Could you check a few things on this model? Use its own coordinates, in mm. Coordinates: 2 decimals unless noted, no trailing zeros. Loops run counter-clockwise (first coordinate to the right, second up) from the corner with the lowest first, then second, coordinate; pieces in that order, holes last. Notation, with made-up numbers: (-25.5, 85) -> (-14.5, 85) arc R6 ccw to (-14.5, 89) -> close; hole circle Ø8 at (-15.75, 24). An arc over 180 degrees is marked (long way). One line per question, with ' | ' between items.
from build123d import *

# Parameters (mm, degrees)
SKETCH1_W               = 48.3
SKETCH1_H               = 44
SKETCH1_R               = 1.6
SKETCH1_R_2             = 2.5527
BOSS_EXTRUDE1_DEPTH     = 6.35
F_1_4_20_TAPPED_HOLE1_D = 5.1054


with BuildPart() as part:
    # Sketch1 → Boss-Extrude1 (new body)
    with BuildSketch(Plane.XY):
        with Locations((24.15, -22)):
            Rectangle(SKETCH1_W, SKETCH1_H)
        with Locations((7.5, -37)):
            Circle(SKETCH1_R, mode=Mode.SUBTRACT)
        with Locations((22.5, -9.3)):
            Circle(SKETCH1_R_2, mode=Mode.SUBTRACT)
        with Locations((35.2, -22)):
            Circle(SKETCH1_R_2, mode=Mode.SUBTRACT)
        with Locations((9.8, -22)):
            Circle(SKETCH1_R_2, mode=Mode.SUBTRACT)
        with Locations((22.5, -34.7)):
            Circle(SKETCH1_R_2, mode=Mode.SUBTRACT)
        with Locations((37.5, -37)):
            Circle(SKETCH1_R, mode=Mode.SUBTRACT)
        with Locations((37.5, -7)):
            Circle(SKETCH1_R, mode=Mode.SUBTRACT)
        with Locations((7.5, -7)):
            Circle(SKETCH1_R, mode=Mode.SUBTRACT)
    extrude(amount=BOSS_EXTRUDE1_DEPTH)

    # 1/4-20 Tapped Hole1 (through all)
    with Locations(Plane(origin=(22.5, -9.3, 6.35), x_dir=(1, 0, 0), z_dir=(0, 0, 1))):
        with Locations((0, 0), (12.7, -12.7), (-12.7, -12.7), (0, -25.4)):
            Hole(F_1_4_20_TAPPED_HOLE1_D / 2)


solid = part.part
1) We'd pull the mould along Z, two halves only. Please class faces 1 (the face through (24, -22, 6.35)), 2 (the face through (24, -22, 0)), 3 (the face through (37.15, -8.56, 3.13)): pulls with the +Z half, pulls with the -Z half, needs draft (parallel to the pull), parting line crosses it, or undercut.
Data:
face 1: pulls with the +Z half | face 2: pulls with the -Z half | face 3: needs draft
2) If we section it at A-A on x = 22.5: Please give me the cut outline in (y, z), and give its area (3 significant figures).
Data:
outline: (-44, 0) -> (-37.25, 0) -> (-37.25, 6.35) -> (-44, 6.35) -> close; (-32.15, 0) -> (-11.85, 0) -> (-11.85, 6.35) -> (-32.15, 6.35) -> close; (-6.75, 0) -> (0, 0) -> (0, 6.35) -> (-6.75, 6.35) -> close | area: 215 mm²
3) I need wall thicknesses on line 1 along Y through (x, z) = (22.5, 3.75); line 2 along X through (y, z) = (-22, 4.5); line 3 along Y through (x, z) = (35.2, 4.25). Which ranges of each line are inside material? Lowest first, please. Write a range as from..to.
Data:
line 1: -44..-37.25, -32.15..-11.85, -6.75..0 | line 2: 0..7.25, 12.35..32.65, 37.75..48.3 | line 3: -44..-24.55, -19.45..0
4) If we section it at B-B on y = -34.7: Please give me the cut outline in (x, z), and give its area (3 significant figures).
Data:
outline: (0, 0) -> (19.95, 0) -> (19.95, 6.35) -> (0, 6.35) -> close; (25.05, 0) -> (48.3, 0) -> (48.3, 6.35) -> (25.05, 6.35) -> close | area: 274 mm²
5) If we section it at D-D on x = 35.2: Please give me the cut outline in (y, z).
Data:
outline: (-44, 0) -> (-24.55, 0) -> (-24.55, 6.35) -> (-44, 6.35) -> close; (-19.45, 0) -> (0, 0) -> (0, 6.35) -> (-19.45, 6.35) -> close
6) If we section it at C-C on z = 3: Give the number of separate pieces and of enclosed holes in the cut face, and give its area (3 significant figures).
Data:
separate pieces: 1 | enclosed holes: 8 | area: 2,010 mm²
